Geometry: final body of the model. Coordinates: model frame, mm. A direction names the side the tool comes from. Coordinates: 2 decimals unless noted, no trailing zeros. Loops run counter-clockwise (first coordinate to the right, second up) from the corner with the lowest first, then second, coordinate; pieces in that order, holes last. Notation, with made-up numbers: (23.25, -35.5) - (34.25, -35.5) arc R19 cw to (34.25, -22.5) - close; hole circle Ø7 at (48.5, 81). An arc over 180 degrees is marked (long way). Answer in a Markdown table with one row per item.
from build123d import *

# Parameters (mm, degrees)
SKETCH1_R           = 1.5
BOSS_EXTRUDE1_DEPTH = 3
CHAMFER1_SIZE       = 3


with BuildPart() as part:
    # Sketch1 → Boss-Extrude1 (new body)
    with BuildSketch(Plane(origin=(0, 0, 0), x_dir=(1, 0, 0), z_dir=(0, 1, 0))):
        Polygon((0, 0), (0, -365), (302.93, -365), (302.93, 0), (230, 0), (230, -201.465), (166.465, -265), (136.465, -265), (72.93, -201.465), (72.93, 0), align=None)
        with Locations(Location((3.97, -328.99, 0), (0, 0, 270))):
            Circle(SKETCH1_R, mode=Mode.SUBTRACT)
        with Locations(Location((68.96, -328.99, 0), (0, 0, 270))):
            Circle(SKETCH1_R, mode=Mode.SUBTRACT)
        with BuildLine():
            Line((26.803641974, -254.267576658), (64.99, -282.415618293))
            Line((64.99, -282.415618293), (64.99, -328.99))
            ThreePointArc((64.99, -328.99), (65.508913215, -330.952371015), (66.93, -332.401744422))
            Line((66.93, -332.401744422), (66.93, -359))
            Line((66.93, -359), (6, -359))
            Line((6, -359), (6, -332.401744422))
            ThreePointArc((6, -332.401744422), (7.421086785, -330.952371015), (7.94, -328.99))
            Line((7.94, -328.99), (7.94, -281.645279056))
            Line((7.94, -281.645279056), (26.803641974, -254.267576658))
        make_face(mode=Mode.SUBTRACT)
        with Locations(Location((3.97, -280.41, 0), (0, 0, 270))):
            Circle(SKETCH1_R, mode=Mode.SUBTRACT)
        with Locations(Location((126.465, -330.25, 0), (0, 0, 270))):
            Circle(SKETCH1_R, mode=Mode.SUBTRACT)
        with BuildLine():
            ThreePointArc((133.965, -322.5), (126.465, -315), (133.965, -307.5))
            Line((133.965, -307.5), (168.965, -307.5))
            ThreePointArc((168.965, -307.5), (176.465, -315), (168.965, -322.5))
            Line((168.965, -322.5), (133.965, -322.5))
        make_face(mode=Mode.SUBTRACT)
        with Locations(Location((126.465, -299.75, 0), (0, 0, 270))):
            Circle(SKETCH1_R, mode=Mode.SUBTRACT)
        with Locations(Location((25.86, -248.64, 0), (0, 0, 270))):
            Circle(SKETCH1_R, mode=Mode.SUBTRACT)
        with Locations(Location((25.86, -190.57, 0), (0, 0, 270))):
            Circle(SKETCH1_R, mode=Mode.SUBTRACT)
        with Locations(Location((176.465, -330.25, 0), (0, 0, 270))):
            Circle(SKETCH1_R, mode=Mode.SUBTRACT)
        with Locations(Location((191.465, -344.035, 0), (0, 0, 270))):
            Circle(SKETCH1_R, mode=Mode.SUBTRACT)
        with Locations(Location((176.465, -299.75, 0), (0, 0, 270))):
            Circle(SKETCH1_R, mode=Mode.SUBTRACT)
        with Locations(Location((191.465, -285.965, 0), (0, 0, 270))):
            Circle(SKETCH1_R, mode=Mode.SUBTRACT)
        with Locations(Location((233.97, -328.99, 0), (0, 0, 270))):
            Circle(SKETCH1_R, mode=Mode.SUBTRACT)
        with Locations(Location((298.96, -328.99, 0), (0, 0, 270))):
            Circle(SKETCH1_R, mode=Mode.SUBTRACT)
        with Locations(Location((233.97, -280.41, 0), (0, 0, 270))):
            Circle(SKETCH1_R, mode=Mode.SUBTRACT)
        with Locations(Location((298.96, -280.41, 0), (0, 0, 270))):
            Circle(SKETCH1_R, mode=Mode.SUBTRACT)
        with Locations(Location((277.07, -248.64, 0), (0, 0, 270))):
            Circle(SKETCH1_R, mode=Mode.SUBTRACT)
        with Locations(Location((277.07, -190.57, 0), (0, 0, 270))):
            Circle(SKETCH1_R, mode=Mode.SUBTRACT)
        with Locations(Location((25.86, -174.43, 0), (0, 0, 270))):
            Circle(SKETCH1_R, mode=Mode.SUBTRACT)
        with BuildLine():
            Line((66.93, -91.018356112), (66.93, -273.981643888))
            Line((66.93, -273.981643888), (31.310895985, -247.725984153))
            Line((31.310895985, -247.725984153), (29.129132873, -250.892480912))
            ThreePointArc((29.129132873, -250.892480912), (29.650735912, -249.819500423), (29.83, -248.64))
            Line((29.83, -248.64), (29.83, -246.634381707))
            Line((29.83, -246.634381707), (28.215581853, -245.444357008))
            ThreePointArc((28.215581853, -245.444357008), (22.664357008, -246.284418147), (23.504418147, -251.835642992))
            Line((23.504418147, -251.835642992), (20.948445099, -249.951576548))
            Line((20.948445099, -249.951576548), (6, -270.774610859))
            Line((6, -270.774610859), (6, -94.53336494))
            Line((6, -94.53336494), (21.89, -117.595279056))
            Line((21.89, -117.595279056), (21.89, -240.781625326))
            Line((21.89, -240.781625326), (24.979472521, -243.058946487))
            Line((24.979472521, -243.058946487), (29.83, -236.302210288))
            Line((29.83, -236.302210288), (29.83, -118.365618293))
            Line((29.83, -118.365618293), (66.93, -91.018356112))
        make_face(mode=Mode.SUBTRACT)
        with Locations(Location((25.86, -116.36, 0), (0, 0, 270))):
            Circle(SKETCH1_R, mode=Mode.SUBTRACT)
        with Locations(Location((3.97, -84.59, 0), (0, 0, 270))):
            Circle(SKETCH1_R, mode=Mode.SUBTRACT)
        with BuildLine():
            Line((64.99, -82.584381707), (26.803641974, -110.732423342))
            Line((26.803641974, -110.732423342), (7.94, -83.354720944))
            Line((7.94, -83.354720944), (7.94, -36.01))
            ThreePointArc((7.94, -36.01), (7.421086785, -34.047628985), (6, -32.598255578))
            Line((6, -32.598255578), (6, -6))
            Line((6, -6), (66.93, -6))
            Line((66.93, -6), (66.93, -32.598255578))
            ThreePointArc((66.93, -32.598255578), (65.508913215, -34.047628985), (64.99, -36.01))
            Line((64.99, -36.01), (64.99, -82.584381707))
        make_face(mode=Mode.SUBTRACT)
        with Locations(Location((68.96, -84.59, 0), (0, 0, 270))):
            Circle(SKETCH1_R, mode=Mode.SUBTRACT)
        with Locations(Location((3.97, -36.01, 0), (0, 0, 270))):
            Circle(SKETCH1_R, mode=Mode.SUBTRACT)
        with Locations(Location((68.96, -36.01, 0), (0, 0, 270))):
            Circle(SKETCH1_R, mode=Mode.SUBTRACT)
        with Locations(Location((277.07, -174.43, 0), (0, 0, 270))):
            Circle(SKETCH1_R, mode=Mode.SUBTRACT)
        with Locations(Location((277.07, -116.36, 0), (0, 0, 270))):
            Circle(SKETCH1_R, mode=Mode.SUBTRACT)
        with Locations(Location((233.97, -84.59, 0), (0, 0, 270))):
            Circle(SKETCH1_R, mode=Mode.SUBTRACT)
        with Locations(Location((298.96, -84.59, 0), (0, 0, 270))):
            Circle(SKETCH1_R, mode=Mode.SUBTRACT)
        with Locations(Location((233.97, -36.01, 0), (0, 0, 270))):
            Circle(SKETCH1_R, mode=Mode.SUBTRACT)
        with Locations(Location((298.96, -36.01, 0), (0, 0, 270))):
            Circle(SKETCH1_R, mode=Mode.SUBTRACT)
        with Locations(Location((68.96, -280.41, 0), (0, 0, 270))):
            Circle(SKETCH1_R, mode=Mode.SUBTRACT)
    extrude(amount=BOSS_EXTRUDE1_DEPTH)

    # Chamfer1
    chamfer1_edges = [part.edges().sort_by_distance(p)[0] for p in [
        (72.93, 1.5, 0),
        (230, 1.5, 0),
        (302.93, 1.5, 0),
        (302.93, 1.5, 365),
        (0, 1.5, 365),
        (0, 1.5, 0),
    ]]
    chamfer(chamfer1_edges, length=CHAMFER1_SIZE)


solid = part.part
(1) Cut plane A-A on z = 261. Output: boundary loops of the cut face in (x, y) (3 decimals).
Verdict:
| item | result |
|---|---|
| outline | (0, 0) - (6, 0) - (6, 3) - (0, 3) - close; (13.017, 0) - (22.165, 0) - (22.165, 3) - (13.017, 3) - close; (35.937, 0) - (49.319, 0) - (49.319, 3) - (35.937, 3) - close; (66.93, 0) - (132.465, 0) - (132.465, 3) - (66.93, 3) - close; (170.465, 0) - (302.93, 0) - (302.93, 3) - (170.465, 3) - close |
(2) Cut plane C-C on y = 1.9. State how many separate pieces and enclosed holes the cut face has, then the cut area to 3 significant figures.
Verdict:
| item | result |
|---|---|
| separate pieces | 1 |
| enclosed holes | 34 |
| area | 53,200 mm² |
(3) Pull-direction query (X, two-part tool) for faces 1 (the face through (126.467, 1.479, 315.165)), 2 (the face through (48.1, 1.5, 104.9)), 3 (the face through (217, 3, 221)); classes: pulls with the +X half, pulls with the -X half, needs draft (parallel to the pull), parting line crosses it, or undercut.
Verdict:
| item | result |
|---|---|
| face 1 | undercut |
| face 2 | undercut |
| face 3 | needs draft |
(4) Cut plane D-D on x = 101.5. Output: boundary loops of the cut face in (y, z) (3 decimals).
Verdict:
| item | result |
|---|---|
| outline | (0, 230.035) - (3, 230.035) - (3, 365) - (0, 365) - close |
(5) Access query for faces 4 (the face through (176.463, 1.479, 314.835)), 5 (the face through (217, 0, 221)), 6 (the face through (105.142, 1.479, 233.677)). Directions: +Z, -Z, +X, -X, +Y, -Y. A direction counts if a zero-diameter tool reaches every point of the face in a straight line with its end or side. Return the directions, or none.
Verdict:
| item | result |
|---|---|
| face 4 | +Y, -Y |
| face 5 | +Z, -Z, +X, -X, -Y |
| face 6 | -Z, +Y, -Y |
(6) Ray query, probe 1 along X at (y, z) = (1.95, 75); probe 2 along X at (y, z) = (0.75, 180); probe 3 along Z at (x, y) = (298.96, 2.35). Return the intervals inside material, ascending.
Verdict:
| item | result |
|---|---|
| probe 1 | x = 0 to 7.94, 64.99 to 72.93, 230 to 302.93 |
| probe 2 | x = 0 to 6, 21.89 to 29.83, 66.93 to 72.93, 230 to 302.93 |
| probe 3 | z = 0 to 34.51, 37.51 to 83.09, 86.09 to 278.91, 281.91 to 327.49, 330.49 to 365 |
(7) Cut plane B-B on z = 318.5. Output: boundary loops of the cut face in (x, y), then the cut area to 3 significant figures.
Verdict:
| item | result |
|---|---|
| outline | (0, 0) - (7.94, 0) - (7.94, 3) - (0, 3) - close; (64.99, 0) - (127.33, 0) - (127.33, 3) - (64.99, 3) - close; (175.6, 0) - (302.93, 0) - (302.93, 3) - (175.6, 3) - close |
| area | 593 mm² |
